Here's the drawing with two shaded views (mm, measured from the low corner). I have some questions. Coordinates: 2 decimals unless noted, no trailing zeros. Write each loop counter-clockwise with the first axis right and the second up, starting at its lowest first coordinate (ties: lowest second). Pieces come first, ordered by that corner, then holes.
Item 1: If we section it at D-D (z = 16.5): Please give me the cut outline in (x, y).
Item 2: We'd pull the mould along Y, two halves only. Please class the marked faces 1, 2 and 3: +Y half, -Y half, draft (parallel to the pull), parting line (faces both ways), or undercut.
Item 3: If we section it at B-B (z = 10.5): Please give me the cut outline in (x, y), then the cut area to 3 significant figures.
Item 4: If I drill on line 1 (X direction, y = 20.25, z = 2); line 2 (Y direction, x = 13.25, z = 10.5); line 3 (Y direction, x = 16, z = 10.5), over which ranges is the centre line in solid material (lowest first)?
Item 5: If we section it at A-A (x = 10.5): Please give me the cut outline in (y, z), then the cut area to 3 significant figures.
Item 6: I'm going to push a flat-ended pin straight in: pin 1 Ø7 at (x, y) = (10.5, 20) entering from +Z. Where does the tip first touch, or does it pass through?
Item 7: If we section it at C-C (y = 20): Please give me the cut outline in (x, z).
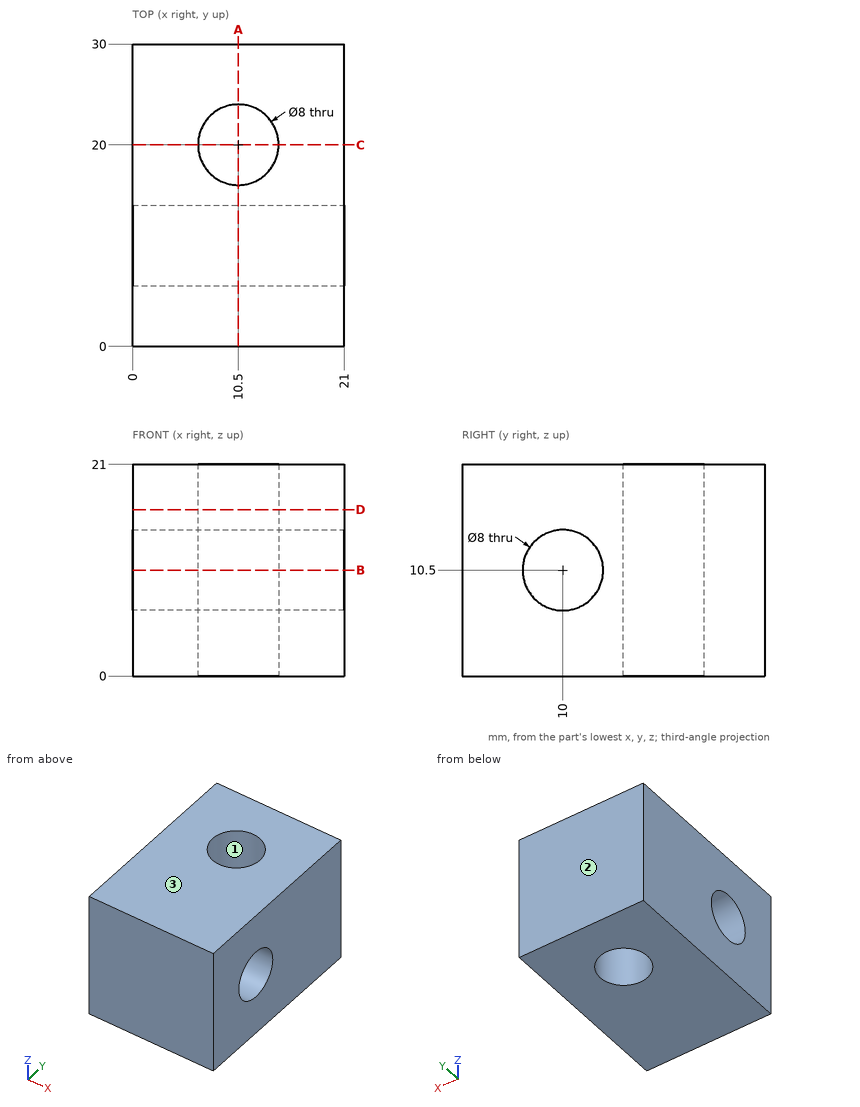
Answer list:
1. outline: (0, 0) - (21, 0) - (21, 30) - (0, 30) - close; hole circle Ø8 at (10.5, 20)
2. face 1: undercut
2. face 2: +Y half
2. face 3: draft
3. outline: (0, 0) - (21, 0) - (21, 6) - (0, 6) - close; (0, 14) - (21, 14) - (21, 30) - (0, 30) - close; hole circle Ø8 at (10.5, 20)
3. area: 412 mm2
4. line 1: x = 0 to 6.51, 14.49 to 21
4. line 2: y = 0 to 6, 14 to 17.1, 22.9 to 30
4. line 3: y = 0 to 6, 14 to 30
5. outline: (0, 0) - (16, 0) - (16, 21) - (0, 21) - close; (24, 0) - (30, 0) - (30, 21) - (24, 21) - close; hole circle Ø8 at (10, 10.5)
5. area: 412 mm2
6. pin 1: passes through
7. outline: (0, 0) - (6.5, 0) - (6.5, 21) - (0, 21) - close; (14.5, 0) - (21, 0) - (21, 21) - (14.5, 21) - close
